Can you work these out from the model? Positions are in its coordinate system, mm. A direction names the side the tool comes from. Coordinates: 2 decimals unless noted, no trailing zeros. Write each loop counter-clockwise with the first axis right and the second up, starting at its lowest first coordinate (ties: lowest second). Pieces come first, ordered by that corner, then holes. Notation, with made-up numbers: (1, 4) - (29, 4) arc R34 ccw to (29, 39) - close; hole circle Ø3 at (81.25, 17.5). An arc over 180 degrees is marked (long way). Use one line per item in the form item = value. Start each with the question number.
(1) For pin 1 Ø5 at (y, z) = (33.5, 1.5) entering from +X; pin 2 Ø3 at (x, z) = (-9, 5) entering from +Y; pin 3 Ø5 at (y, z) = (32.5, 3.5) entering from -X, each with a flat end and sliding along its axis, tell me the tip position at first contact or that it passes through.
(2) If we section it at A-A on x = 6: Please give me the cut outline in (y, z), then the cut area to 3 significant figures.
(3) If we section it at C-C on y = 11: Please give me the cut outline in (x, z), then the cut area to 3 significant figures.
(4) If we section it at B-B on z = 3.5: Please give me the cut outline in (x, y).
(5) If I drill on probe 1 along Z at (x, y) = (0.95, 38) (3 decimals); probe 2 along Y at (x, z) = (6.75, 1.75); probe 3 along X at (y, z) = (-6, 6), over which ranges is the centre line in solid material (lowest first)? Write a range as from..to.
(6) Thinking about a two-plate mould opening in X: for faces 5 (the face through (-2, 23, 5)), 6 (the face through (0, 0, 5)), 7 (the face through (2, 23, 5)), which applies, pulls with the +X half, pulls with the -X half, needs draft (parallel to the pull), parting line crosses it, or undercut?
(7) If we section it at D-D on z = 0.5: Please give me the cut outline in (x, y).
(8) On a 3-axis mill with a long thin cutter (end or side, diameter ignored), from which of +Z, -Z, +X, -X, +Y, -Y can I reach the whole of each face in a straight line? I mean faces 1 (the face through (-8, 3, 5)), 2 (the face through (11.992, -3, 5)), 3 (the face through (0, 41, 1)), 4 (the face through (9, 3, 5)). Say none if no direction works.
```python
from build123d import *

# Parameters (mm, degrees)
F0_W     = 4
F0_H     = 40
F1_DEPTH = 10
F2_R     = 2.375
F3_DEPTH = 12.5
F4_R     = 4.99999


# Not quite as in the source:
# - a fillet or chamfer is up to 0.001 mm smaller than in the source, because OpenCascade refuses the exact size


with BuildPart() as f1:
    # F0 (on Top) → F1 (new body)
    with BuildSketch(Plane.XY):
        Polygon((-12.0077335707, 3), (-12.0077335707, 0), (11.9922664293, 0), (11.9922664293, -6.25), (14.9922664293, -6.25), (14.9922664293, 3), (2, 3), (-2, 3), align=None)
        Polygon((-12.0077335707, -6.25), (-12.0077335707, 0), (-12.0077335707, 3), (-15.0077335707, 3), (-15.0077335707, -9.25), (-12.0077335707, -9.25), align=None)
        Polygon((11.9922664293, -6.25), (-12.0077335707, -6.25), (-12.0077335707, -9.25), (14.9922664293, -9.25), (14.9922664293, -6.25), align=None)
        with Locations((0, 23)):
            Rectangle(F0_W, F0_H)
    extrude(amount=F1_DEPTH)

    # F2 (on Right) → F3 (cut, symmetric)
    with BuildSketch(Plane.YZ):
        with Locations((38, 5)):
            Circle(F2_R)
    extrude(amount=F3_DEPTH, both=True, mode=Mode.SUBTRACT)

    # F4 (radius 5 in the source; OpenCascade refuses exactly that, so slightly less here)
    f4_edges = [f1.edges().sort_by_distance(p)[0] for p in [
        (0, 43, 10),
        (0, 43, 0),
    ]]
    fillet(f4_edges, radius=F4_R)


solid = f1.part
```
Reported:
q1.pin_1 = 2
q1.pin_2 = 3
q1.pin_3 = -2
q2.outline = (-9.25, 0) - (-6.25, 0) - (-6.25, 10) - (-9.25, 10) - close; (0, 0) - (3, 0) - (3, 10) - (0, 10) - close
q2.area = 60.0 mm2
q3.outline = (-2, 0) - (2, 0) - (2, 10) - (-2, 10) - close
q3.area = 40.0 mm2
q4.outline = (-15.01, -9.25) - (14.99, -9.25) - (14.99, 3) - (2, 3) - (2, 36.16) - (-2, 36.16) - (-2, 3) - (-15.01, 3) - close; (-2, 39.84) - (2, 39.84) - (2, 42.77) - (-2, 42.77) - close; hole (-12.01, -6.25) - (11.99, -6.25) - (11.99, 0) - (-12.01, 0) - close
q5.probe_1 = 0..2.625, 7.375..10
q5.probe_2 = -9.25..-6.25, 0..3
q5.probe_3 = -15.01..-12.01, 11.99..14.99
q6.face_5 = pulls with the -X half
q6.face_6 = undercut
q6.face_7 = pulls with the +X half
q7.outline = (-15.01, -9.25) - (14.99, -9.25) - (14.99, 3) - (2, 3) - (2, 40.18) - (-2, 40.18) - (-2, 3) - (-15.01, 3) - close; hole (-12.01, -6.25) - (11.99, -6.25) - (11.99, 0) - (-12.01, 0) - close
q8.face_1 = +Z, -Z, -X, +Y
q8.face_2 = +Z, -Z
q8.face_3 = -Z, +X, -X, +Y
q8.face_4 = +Z, -Z, +X, +Y
